```python
from build123d import *

# Parameters (mm, degrees)
MODEL_R             = 1
MODEL_R_2           = 1.5
MODEL_W             = 31.2
MODEL_H             = 31.2
MODEL_W_2           = 12
MODEL_H_2           = 5
MODEL_W_3           = 43.5
MODEL_H_3           = 38
BOSS_EXTRUDE1_DEPTH = 3


with BuildPart() as part:
    # Model → Boss-Extrude1 (new body)
    with BuildSketch(Plane.XY):
        Polygon((-155.141927583, -53.052781364), (-152.141927583, -53.052781364), (-152.141927583, -23.052781364), (-155.141927583, -23.052781364), (-155.141927583, 6.947218636), (-147.141927583, 6.947218636), (-147.141927583, 3.947218636), (-137.141927583, 3.947218636), (-137.141927583, 6.947218636), (-73.641927583, 6.947218636), (-73.641927583, 3.947218636), (-53.641927583, 3.947218636), (-53.641927583, 6.947218636), (6.858072417, 6.947218636), (6.858072417, 3.947218636), (16.858072417, 3.947218636), (16.858072417, 6.947218636), (24.858072417, 6.947218636), (24.858072417, -23.052781364), (27.858072417, -23.052781364), (27.858072417, -53.052781364), (24.858072417, -53.052781364), (24.858072417, -83.052781364), (-48.641927583, -83.052781364), (-48.641927583, -82.052781364), (-78.641927583, -82.052781364), (-78.641927583, -83.052781364), (-155.141927583, -83.052781364), align=None)
        with Locations((-145.091927583, -50.925083063)):
            Circle(MODEL_R, mode=Mode.SUBTRACT)
        with Locations((-115.091927583, -50.925083063)):
            Circle(MODEL_R, mode=Mode.SUBTRACT)
        with Locations((17.808072417, -65.052781364)):
            Circle(MODEL_R, mode=Mode.SUBTRACT)
        with Locations((-12.191927583, -65.052781364)):
            Circle(MODEL_R, mode=Mode.SUBTRACT)
        with Locations((-108.141927583, -24.052781364)):
            Circle(MODEL_R_2, mode=Mode.SUBTRACT)
        with Locations((-56.141927583, -24.052781364)):
            Circle(MODEL_R_2, mode=Mode.SUBTRACT)
        with Locations((-56.141927583, -56.052781364)):
            Circle(MODEL_R_2, mode=Mode.SUBTRACT)
        with Locations((-108.141927583, -56.052781364)):
            Circle(MODEL_R_2, mode=Mode.SUBTRACT)
        with Locations((17.808072417, -72.052781364)):
            Circle(MODEL_R, mode=Mode.SUBTRACT)
        with Locations((17.808072417, -58.052781364)):
            Circle(MODEL_R, mode=Mode.SUBTRACT)
        with Locations((-145.091927583, -43.925083063)):
            Circle(MODEL_R, mode=Mode.SUBTRACT)
        with Locations((-145.091927583, -57.925083063)):
            Circle(MODEL_R, mode=Mode.SUBTRACT)
        with Locations((-40.141927583, -26.052781364)):
            Circle(MODEL_R, mode=Mode.SUBTRACT)
        with Locations((14.858072417, -26.052781364)):
            Circle(MODEL_R, mode=Mode.SUBTRACT)
        with Locations((-40.141927583, -3.052781364)):
            Circle(MODEL_R, mode=Mode.SUBTRACT)
        with Locations((14.858072417, -3.052781364)):
            Circle(MODEL_R, mode=Mode.SUBTRACT)
        with Locations((-131.541927583, -19.325083063)):
            Rectangle(MODEL_W, MODEL_H, mode=Mode.SUBTRACT)
        with Locations((18.858072417, -41.552781364)):
            Rectangle(MODEL_W_2, MODEL_H_2, mode=Mode.SUBTRACT)
        with Locations((-82.891927583, -40.052781364)):
            Rectangle(MODEL_W_3, MODEL_H_3, mode=Mode.SUBTRACT)
    extrude(amount=BOSS_EXTRUDE1_DEPTH)


solid = part.part
```
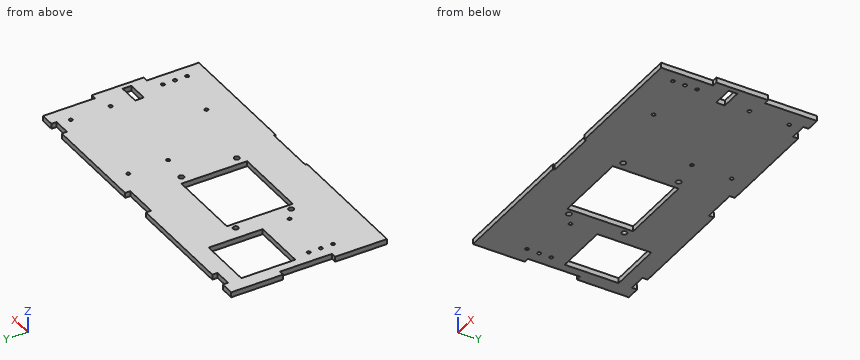
Geometry check sheet. Reference: the model listing, model coordinates, mm. Round coordinates to 2 decimals unless told otherwise and drop trailing zeros. Loops run counter-clockwise (first coordinate to the right, second up) from the corner with the lowest first, then second, coordinate; pieces in that order, holes last. Notation, with made-up numbers: (28, -33.75) -> (32, -33.75) arc R32 cw to (32, -5.75) -> close; hole circle Ø11 at (6.25, 78). An arc over 180 degrees is marked (long way). Use a Markdown table: item, result.
(1) Sectioned sample at D-D (z = 2.55). Give the number of separate pieces and of enclosed holes in the cut face, then the cut area to 3 significant figures.
Calculated:
| item | result |
|---|---|
| separate pieces | 1 |
| enclosed holes | 19 |
| area | 13,300 mm² |
(2) Sectioned sample at A-A (x = -130). Enter the section's corners in (y, z).
Calculated:
| item | result |
|---|---|
| outline | (-83.05, 0) -> (-34.93, 0) -> (-34.93, 3) -> (-83.05, 3) -> close; (-3.73, 0) -> (6.95, 0) -> (6.95, 3) -> (-3.73, 3) -> close |
(3) Scan lines: probe 1 along X at (y, z) = (-51, 2.4); probe 2 along Y at (x, z) = (-85.5, 2.4); probe 3 along Y at (x, z) = (-107, 0.25). Record each from-to range of solid material in increasing order.
Calculated:
| item | result |
|---|---|
| probe 1 | -152.14 to -146.09, -144.09 to -116.09, -114.09 to -104.64, -61.14 to 27.86 |
| probe 2 | -83.05 to -59.05, -21.05 to 6.95 |
| probe 3 | -83.05 to -57.03, -55.08 to -25.03, -23.08 to 6.95 |
(4) Sectioned sample at B-B (y = -47.5). Enter the section's corners in (x, z), then the cut area to 4 significant figures.
Calculated:
| item | result |
|---|---|
| outline | (-152.14, 0) -> (-104.64, 0) -> (-104.64, 3) -> (-152.14, 3) -> close; (-61.14, 0) -> (27.86, 0) -> (27.86, 3) -> (-61.14, 3) -> close |
| area | 409.5 mm² |
(5) Go/stop test with flat-tipped pins: P1, Ø3, axis at x = -40.14, y = -26.05, coming from the +Z side; P2, Ø1.6, axis at x = 17.81, y = -65.05, coming from the -Z side; P3, Ø1.5, axis at y = 6, z = 1, coming from the +X side; P4, Ø1.5, axis at x = 13, z = 1, coming from the +Y side. Record where each tip stops, or that it passes through.
Calculated:
| item | result |
|---|---|
| P1 | z = 3 |
| P2 | through |
| P3 | x = 24.86 |
| P4 | y = 3.95 |
(6) Sectioned sample at C-C (y = -32). Enter the section's corners in (x, z), then the cut area to 3 significant figures.
Calculated:
| item | result |
|---|---|
| outline | (-152.14, 0) -> (-147.14, 0) -> (-147.14, 3) -> (-152.14, 3) -> close; (-115.94, 0) -> (-104.64, 0) -> (-104.64, 3) -> (-115.94, 3) -> close; (-61.14, 0) -> (27.86, 0) -> (27.86, 3) -> (-61.14, 3) -> close |
| area | 316 mm² |
